Autodesk Inventor part; units mm, degrees
ref_plane "YZ Plane" through (0, 0, 0) normal (1, 0, 0) x (0, 1, 0)
ref_plane "XZ Plane" through (0, 0, 0) normal (0, 1, 0) x (-1, 0, 0)
ref_plane "XY Plane" through (0, 0, 0) normal (0, 0, 1) x (1, 0, 0)
sketch "Sketch1" plane through (0, 0, 0) normal (0, 1, 0) x (-1, 0, 0)
  line L0 (14.3928, 0) -> (-16, 0) construction
  line L1 (0, 16.4961) -> (0, -25.3301) construction
  circle A0 centre (5, 24.5) radius 1.6
  line L2 (10, 24.5) -> (10, 30)
  line L3 (10, 30) -> (5, 30)
  line L4 (5, 30) -> (0, 30)
  line L5 (0, 30) -> (0, 24.5)
  line L6 (5, 24.5) -> (5, 26.1)
  line L7 (0, 24.5) -> (0, 0)
  line L8 (0, 0) -> (10, 0)
  line L9 (10, 0) -> (10, 24.5)
  circle A1 centre (5, -24.5) radius 1.6
  line L10 (10, -24.5) -> (10, -30)
  line L11 (10, -30) -> (5, -30)
  line L12 (5, -30) -> (0, -30)
  line L13 (0, -30) -> (0, -24.5)
  line L14 (0, -24.5) -> (0, 0)
  line L15 (10, 0) -> (10, -24.5)
  circle A2 centre (-5, 24.5) radius 1.6
  line L16 (-10, 24.5) -> (-10, 30)
  line L17 (-10, 30) -> (-5, 30)
  line L18 (-5, 30) -> (0, 30)
  line L19 (-10, 0) -> (-10, 24.5)
  circle A3 centre (-5, -24.5) radius 1.6
  line L20 (-10, -24.5) -> (-10, -30)
  line L21 (-10, -30) -> (-5, -30)
  line L22 (-5, -30) -> (0, -30)
  line L23 (-10, 0) -> (-10, -24.5)
  line L24 (-10, 30) -> (-8, 30)
  line L25 (-8, 30) -> (-8, -30)
  line L26 (-8, -30) -> (-10, -30)
  line L27 (-10, -30) -> (-10, 30)
  line L28 (10, 30) -> (-10, 30)
  line L29 (-10, 30) -> (-10, 28)
  line L30 (-10, 28) -> (10, 28)
  line L31 (10, 28) -> (10, 30)
  line L32 (-10, -30) -> (10, -30)
  line L33 (10, -30) -> (10, -28)
  line L34 (10, -28) -> (-10, -28)
  line L35 (-10, -28) -> (-10, -30)
  line L36 (-10, -30) -> (-12, -30)
  line L37 (-12, -30) -> (-12, 30)
  line L38 (-12, 30) -> (-10, 30)
  line L39 (-10, 30) -> (-10, -30)
  line L40 (-10, -28) -> (-12, -28)
  line L41 (-10, 28) -> (-12, 28)
  point P0 (5, 27.25)
  point P1 (-8, -28)
  point P2 (-8, 28)
  dimension "d0" = 3.2
  dimension "d2" = 24.5
  dimension "d3" = 5
  dimension "d6" = 2
extrude "Extrusion1" add sketch "Sketch1" along normal blind 3 contours L9 L8 L7 L5 L30 L2 | L15 L10 L34 L13 L14 L8 | L5 L7 L14 L13 L34 L25 L30 | L25 L34 L20 L23 L19 L16 L30
extrude "Extrusion2" add sketch "Sketch1" along normal blind 15 contours L25 L34 L20 L23 L19 L16 L30 | L16 L19 L23 L20 L40 L37 L41
sketch "Sketch2" plane through (8, 3, 30) normal (-1, 0, 0) x (0, 0, 1)
  line L0 (-58, 12) -> (-2, 12)
  line L1 (-30, 12) -> (-30, 0)
  line L2 (-2, 0) -> (-58, 0)
  circle A0 centre (-20, 6) radius 1.6
  circle A1 centre (-20, 6) radius 2.75
  circle A2 centre (-40, 6) radius 1.6
  circle A3 centre (-40, 6) radius 2.75
  point P0 (-30, -3)
  point P1 (-60, 12)
  point P2 (0, 12)
  point P3 (0, 0)
  point P4 (-60, 0)
  dimension "d9" = 3.2
  dimension "d10" = 5.5
  dimension "d13" = 10
extrude "Extrusion3" cut sketch "Sketch2" against normal blind 15 contours A0 | A2
properties part number "Holder Servo Lifter_3DPrint"
Geometry check sheet. Reference: the model listing, model coordinates, mm. A direction names the side the tool comes from. Round coordinates to 2 decimals unless told otherwise and drop trailing zeros. Write each loop counter-clockwise with the first axis right and the second up, starting at its lowest first coordinate (ties: lowest second). Pieces come first, ordered by that corner, then holes. Notation, with made-up numbers: (-7, 69.5) -> (22, 69.5) arc R4 cw to (22, 73.5) -> close; hole circle Ø2 at (10, 54.5). An arc over 180 degrees is marked (long way). One line per item, written item: value. Start each with the question number.
(1) Cross-section at C-C, the plane z = 10. Record the cut outline in (x, y).
(2) Draft check along X on faces 3 (the flat face through (8, 9, 0)), 4 (the cylindrical face through (-4.792, 1.479, 22.914)), 5 (the cylindrical face through (9.97, 8.03, -11.27)). Enter one of: +X half, -X half, draft (parallel to the pull), parting line (faces both ways), or undercut.
(3) Cross-section at B-B, the plane y = 9. Record the cut outline in (x, z), and give its area (3 significant figures).
(4) Cross-section at D-D, the plane z = -24.5. Record the cut outline in (x, y), and give its area (3 significant figures).
(5) Cross-section at A-A, the plane x = -5. Record the cut outline in (y, z).
(6) Scan lines: line 1 (Z direction, x = -5, y = 1.2); line 2 (X direction, y = 7.5, z = -23); line 3 (Y direction, x = 0, z = -10). Record each from-to range of solid material in increasing order. Write a range as [from, to].
(7) Go/stop test with flat-tipped pins: pin 1 Ø12 at (x, z) = (-3.5, -10.5) entering from +Y; pin 2 Ø3.5 at (x, z) = (5, 24.5) entering from -Y; pin 3 Ø3.5 at (y, z) = (12, -10) entering from -X. Record where each tip stops, or that it passes through.
(8) Access from +Z, -Z, +X, -X, +Y, -Y to the whole of each face (thin tool, end or side, straight path). Record for faces 1 (the flat face through (-1, 3, 0)), 2 (the cylindrical face through (5.208, 1.479, -26.086)).
Answer:
1. outline: (-10, 0) -> (12, 0) -> (12, 7.4) -> (8, 7.4) -> (8, 3) -> (-10, 3) -> close; (8, 10.6) -> (12, 10.6) -> (12, 15) -> (8, 15) -> close
2. face 3: -X half
2. face 4: undercut
2. face 5: draft
3. outline: (8, -28) -> (12, -28) -> (12, -11.6) -> (8, -11.6) -> close; (8, -8.4) -> (12, -8.4) -> (12, 8.4) -> (8, 8.4) -> close; (8, 11.6) -> (12, 11.6) -> (12, 28) -> (8, 28) -> close
3. area: 198 mm²
4. outline: (-10, 0) -> (-6.6, 0) -> (-6.6, 3) -> (-10, 3) -> close; (-3.4, 0) -> (3.4, 0) -> (3.4, 3) -> (-3.4, 3) -> close; (6.6, 0) -> (12, 0) -> (12, 15) -> (8, 15) -> (8, 3) -> (6.6, 3) -> close
4. area: 94.8 mm²
5. outline: (0, -28) -> (3, -28) -> (3, -26.1) -> (0, -26.1) -> close; (0, -22.9) -> (3, -22.9) -> (3, 22.9) -> (0, 22.9) -> close; (0, 26.1) -> (3, 26.1) -> (3, 28) -> (0, 28) -> close
6. line 1: [-28, -26.1], [-22.9, 22.9], [26.1, 28]
6. line 2: [8, 12]
6. line 3: [0, 3]
7. pin 1: y = 3
7. pin 2: y = 0
7. pin 3: x = 8
8. face 1: +Z, -Z, -X, +Y
8. face 2: +Y, -Y
